Design review of the part built by this model. Coordinates are the model's own, in mm. Coordinates: 2 decimals unless noted, no trailing zeros. Loops run counter-clockwise (first coordinate to the right, second up) from the corner with the lowest first, then second, coordinate; pieces in that order, holes last. Notation, with made-up numbers: M 81,82.25 L 88,82.25 A12 cw 88,92.25 Z; hole C 38.25,67 d5. An arc over 180 degrees is marked long. Put each result on its own line as item: value. Start each with the question number.
(1) Clearance check with flat-ended pins moving along their axes: pin 1 (1 mm diameter, centred on y = -30, z = 27.5, fed in from +X); pin 2 (1.5 mm diameter, centred on y = -173, z = 29.5, fed in from -X); pin 3 (8 mm diameter, centred on x = 11, y = -199.5, fed in from +Z). State where each tip first meets the part, or that it passes through.
(2) For probe 1 along Y at (x, z) = (-33, -7); probe 2 along Y at (x, z) = (39, -35.5); probe 3 along Z at (x, y) = (-28, -71), list the stretches that pass through material, from the lowest coordinate up. Write a range as [from, to].
(3) Take a section at A-A, the plane y = -115.5. Give the boundary of the cut face in (x, z).
(4) Take a section at B-B, the plane y = -17.5. Give the boundary of the cut face in (x, z).
```python
from build123d import *

# Parameters (mm, degrees)
F1_DEPTH = 228.6
F2_R     = 22.86
F3_R     = 25.4


with BuildPart() as f1:
    # F0 (on Front) → F1 (new body)
    with BuildSketch(Plane.XZ):
        Polygon((-34.895125, 54.553078), (-64.408069, 6.731181), (-45.420423, -46.159433), (7.769728, -64.291052), (55.109115, -34.010198), (60.950214, 21.881029), (20.89456, 61.295395), align=None)
    extrude(amount=F1_DEPTH)

    # F2
    f2_edges = [f1.edges().sort_by_distance(p)[0] for p in [
        (-7.000283, -228.6, 57.924237),
        (-49.651597, -228.6, 30.642129),
        (-54.914246, -228.6, -19.714126),
        (-18.825348, -228.6, -55.225243),
        (31.439421, -228.6, -49.150625),
        (58.029665, -228.6, -6.064584),
        (40.922387, -228.6, 41.588212),
    ]]
    fillet(f2_edges, radius=F2_R)

    # F3
    f3_edges = [f1.edges().sort_by_distance(p)[0] for p in [
        (-7.000283, 0, 57.924237),
        (-49.651597, 0, 30.642129),
        (-54.914246, 0, -19.714126),
        (-18.825348, 0, -55.225243),
        (31.439421, 0, -49.150625),
        (58.029665, 0, -6.064584),
        (40.922387, 0, 41.588212),
    ]]
    fillet(f3_edges, radius=F3_R)


solid = f1.part
```
Computed values:
1. pin 1: stops at x = 55.75
1. pin 2: stops at x = -50.82
1. pin 3: stops at z = 60.58
2. probe 1: y = [-228.6, 0]
2. probe 2: y = [-222.6, -7.45]
2. probe 3: z = [-52.1, 55.39]
3. outline: M -64.41,6.73 L -45.42,-46.16 L 7.77,-64.29 L 55.11,-34.01 L 60.95,21.88 L 20.89,61.3 L -34.9,54.55 Z
4. outline: M -63.02,6.59 L -44.44,-45.16 L 7.6,-62.9 L 53.92,-33.28 L 59.63,21.41 L 20.44,59.97 L -34.14,53.38 Z
